The model under review builds one solid part; all positions refer to its coordinate system, in mm. A direction names the side the tool comes from. Round coordinates to 2 decimals unless told otherwise and drop trailing zeros. Write each loop counter-clockwise with the first axis right and the second up, starting at its lowest first coordinate (ties: lowest second). Pieces come first, ordered by that corner, then holes. Notation, with made-up numbers: (-7.5, 26.5) - (51.5, 26.5) arc R21 cw to (51.5, 36.5) - close; hole circle Ø10 at (31, -28). An arc over 180 degrees is marked (long way). Write each question's results on one line, items separated by ' | '.
```python
from build123d import *

# Parameters (mm, degrees)
SKETCH1_W           = 180
SKETCH1_H           = 80
SKETCH1_R           = 1.5
BOSS_EXTRUDE1_DEPTH = 4
SKETCH2_W           = 4
SKETCH2_H           = 24
SKETCH2_H_2         = 15.4
CUT_EXTRUDE1_DEPTH  = 4


with BuildPart() as part:
    # Sketch1 → Boss-Extrude1 (new body)
    with BuildSketch(Plane.XY):
        with Locations((2.700642055, -21.117125984)):
            Rectangle(SKETCH1_W, SKETCH1_H)
        with Locations((-77.299357945, -9.617125984)):
            Circle(SKETCH1_R, mode=Mode.SUBTRACT)
        with Locations((82.700642055, -9.617125984)):
            Circle(SKETCH1_R, mode=Mode.SUBTRACT)
        with Locations((61.700642055, -51.117125984)):
            Circle(SKETCH1_R, mode=Mode.SUBTRACT)
        with Locations((-56.299357945, -51.117125984)):
            Circle(SKETCH1_R, mode=Mode.SUBTRACT)
    extrude(amount=BOSS_EXTRUDE1_DEPTH)

    # Sketch2 → Cut-Extrude1 (cut)
    with BuildSketch(Plane.XY.offset(4)):
        with Locations((-4.799357945, -13.117125984)):
            Rectangle(SKETCH2_W, SKETCH2_H)
        with Locations((2.700642055, -8.817125984)):
            Rectangle(SKETCH2_W, SKETCH2_H_2)
        with Locations((10.200642055, -13.117125984)):
            Rectangle(SKETCH2_W, SKETCH2_H)
    extrude(amount=-CUT_EXTRUDE1_DEPTH, mode=Mode.SUBTRACT)


solid = part.part
```
Q1. We need section A-A (z = 3.25). State the section outline as (x, y) points, plus the area to 3 significant figures.
Evaluation:
outline: (-87.3, -61.12) - (92.7, -61.12) - (92.7, 18.88) - (-87.3, 18.88) - close; hole circle Ø3 at (-77.3, -9.62); hole circle Ø3 at (-56.3, -51.12); hole (-6.8, -25.12) - (-2.8, -25.12) - (-2.8, -1.12) - (-6.8, -1.12) - close; hole (0.7, -16.52) - (4.7, -16.52) - (4.7, -1.12) - (0.7, -1.12) - close; hole (8.2, -25.12) - (12.2, -25.12) - (12.2, -1.12) - (8.2, -1.12) - close; hole circle Ø3 at (61.7, -51.12); hole circle Ø3 at (82.7, -9.62) | area: 14,100 mm^2
Q2. Tool access review of faces 5 (the flat face through (10, -1.117, 2)), 6 (the flat face through (-87.299, -22, 2)): name each direction out of +Z, -Z, +X, -X, +Y, -Y from which nothing blocks a thin tool from reaching the whole face with its end or side.
Evaluation:
face 5: +Z, -Z | face 6: +Z, -Z, -X, +Y, -Y
Q3. The part is to be moulded in two halves that separate along Y. For faces 1 (the flat face through (-5, -25.117, 2)), 2 (the flat face through (92.701, -22, 2)), 3 (the flat face through (4.701, -9, 2)), 4 (the flat face through (1, -61.117, 2)), say which applies: released by +Y, released by -Y, zero draft, split by the parting line, or undercut.
Evaluation:
face 1: undercut | face 2: zero draft | face 3: undercut | face 4: released by -Y
Q4. For probe 1 along X at (y, z) = (-6.5, 1.1); probe 2 along X at (y, z) = (-25, 1.4); probe 3 along Y at (x, z) = (4, 1.45), list the stretches that pass through material, from the lowest coordinate up.
Evaluation:
probe 1: x = -87.3 to -6.8, -2.8 to 0.7, 4.7 to 8.2, 12.2 to 92.7 | probe 2: x = -87.3 to -6.8, -2.8 to 8.2, 12.2 to 92.7 | probe 3: y = -61.12 to -16.52, -1.12 to 18.88
